Autodesk Inventor part; units mm, degrees
ref_plane "Work Plane1" through (0, 99.5, 0) normal (0, 1, 0) x (1, 0, 0)
ref_plane "Work Plane2" through (0, 0.5, 0) normal (0, -1, 0) x (1, 0, 0)
ref_plane "YZ Plane" through (0, 0, 0) normal (1, 0, 0) x (0, 1, 0)
sketch "Sketch1" plane through (0, 0, 0) normal (0, 1, 0) x (-1, 0, 0)
  circle A0 centre (0, 0) radius 1.4
  dimension "d0" = 2.8
extrude "Extrusion1" add sketch "Sketch1" along normal blind 100
ref_plane "Work Plane1" through (0, 99.5, 0) normal (0, 1, 0) x (1, 0, 0)
sketch "Sketch2" plane through (0, 99.5, 0) normal (0, 1, 0) x (1, 0, 0)
  line L0 (0, 0) -> (0, -1.5)
  line L1 (0, 0) -> (0, 1.5)
  dimension "d4" = 1.5
  dimension "d5" = 1.5
sketch "Sketch3" plane through (0, 0, 0) normal (1, 0, 0) x (0, 1, 0)
  line L0 (99.5, 0) -> (99.5, 1.5)
  line L1 (99.5, 0) -> (99.5, -1.5)
  line L2 (99.5, 1.5) -> (100.5, 1.5)
  line L3 (100.5, 1.5) -> (100.5, -1.5)
  line L4 (100.5, -1.5) -> (99.5, -1.5)
  line L5 (102, 1.659) -> (102, -3.2084)
  point P0 (0, 0)
  dimension "d6" = 1
  dimension "d7" = 2.5
revolve "Revolution1" add sketch "Sketch3" angle 360 about axis through (0, 102, 1.659) along (0, 0, -1)
ref_plane "Work Plane2" through (0, 0.5, 0) normal (0, -1, 0) x (1, 0, 0)
sketch "Sketch4" plane through (0, 0.5, 0) normal (0, -1, 0) x (1, 0, 0)
  line L0 (0, 0) -> (0, -2.1121)
  line L1 (3.5, -0.5) -> (3.5, 0.5)
  line L2 (3.5, 0.5) -> (0, 0.5)
  line L3 (3.5, -0.5) -> (0, -0.5)
  line L4 (-3.5, -0.5) -> (-3.5, 0.5)
  line L5 (-3.5, 0.5) -> (0, 0.5)
  line L6 (-3.5, -0.5) -> (0, -0.5)
  dimension "d12" = 3.5
  dimension "d13" = 1
extrude "Extrusion2" add sketch "Sketch4" along normal blind 9
sketch "Sketch5" plane through (3.5, 0.5, -0.5) normal (0, 0, -1) x (-1, 0, 0)
  line L0 (3.5, -0.5) -> (3.5, -9)
  line L1 (7, -9) -> (0, -9)
  line L2 (3.5, -9) -> (3.5, -5.5)
  line L3 (3.5, -9) -> (3.5, -9.0551)
  circle A0 centre (3.5, -5.5) radius 2
  dimension "d16" = 3.5
  dimension "d17" = 4
extrude "Extrusion3" add sketch "Sketch5" along normal blind 1.2
sketch "Sketch6" plane through (-3.5, 0.5, 0.5) normal (0, 0, 1) x (1, 0, 0)
  circle A0 centre (3.5, -5.5) radius 2
  point P0 (3.5, -0.5)
extrude "Extrusion4" add sketch "Sketch6" along normal blind 1.9
properties part number "101-05" material "Aluminum 6061"
CAD build for the part. Positions are in the model's coordinates, mm. A direction names the side the tool comes from. Round coordinates to 2 decimals unless told otherwise and drop trailing zeros. Loops run counter-clockwise (first coordinate to the right, second up) from the corner with the lowest first, then second, coordinate; pieces in that order, holes last. Notation, with made-up numbers: (-1, 53.5) - (18, 53.5) arc R28 ccw to (18, 87.5) - close; hole circle Ø8 at (54.5, 26). An arc over 180 degrees is marked (long way). Return JSON: item names as keys, results as strings. Group by question number.
Q1. Drill centre lines: line 1 along Y through (x, z) = (0, 0.9); line 2 along Y through (x, z) = (0, -0.15); line 3 along X through (y, z) = (102, -0.25). Where is each one in solid material? Low to high. Write a range as [from, to].
Q2. Flat gauge pins, fed straight in: pin 1 Ø2.5 at (x, y) = (-1, 101.5) entering from -Z; pin 2 Ø1.1 at (x, z) = (2.5, 0) entering from +Y; pin 3 Ø2 at (x, z) = (2, 1) entering from +Y. Where does each tip first touch, or does it go through?
Q3. Band-saw the part on A-A on x = 0. Give the cut face in (y, z), plus the area to 4 significant figures.
Q4. Band-saw the part on C-C on y = -5. Give the cut face in (x, z).
Q5. Tool access for faces 4 (the face through (1.4, 49.26, -0.06)), 5 (the face through (0, -7, 1)), 6 (the face through (-1, -3, -0.5)): list every direction of +Z, -Z, +X, -X, +Y, -Y with a clear straight run to the whole face (end or side of a thin tool).
Q6. Band-saw the part on B-B on y = 102. Give the cut face in (x, z), plus the area to 3 significant figures.
Q7. Two-plate mould, pull along X, no slides. Class faces 1 (the face through (-0.1, 104.5, 0)), 2 (the face through (2, 102, 1.5)), 3 (the face through (-1.265, 101.194, -0.021)): +X half, -X half, draft (parallel to the pull), parting line (faces both ways), or undercut.
Solutions:
{
 "1": {"line 1": "y = [-7, -3], [0, 100.5], [103.5, 104.5]", "line 2": "y = [-8.5, 100.5], [103.5, 104.5]", "line 3": "x = [-2.5, -1.5], [1.5, 2.5]"},
 "2": {"pin 1": "stops at z = -1.5", "pin 2": "stops at y = 103.56", "pin 3": "stops at y = 104.29"},
 "3": {"outline": "(-8.5, -0.5) - (-7, -0.5) - (-7, -1.7) - (-3, -1.7) - (-3, -0.5) - (0, -0.5) - (0, -1.4) - (99.5, -1.4) - (99.5, -1.5) - (100.5, -1.5) - (100.5, 1.5) - (99.5, 1.5) - (99.5, 1.4) - (0, 1.4) - (0, 0.5) - (-3, 0.5) - (-3, 2.4) - (-7, 2.4) - (-7, 0.5) - (-8.5, 0.5) - close; (103.5, -1.5) - (104.5, -1.5) - (104.5, 1.5) - (103.5, 1.5) - close", "area": "305.5 mm^2"},
 "4": {"outline": "(-3.5, -0.5) - (-2, -0.5) - (-2, -1.7) - (2, -1.7) - (2, -0.5) - (3.5, -0.5) - (3.5, 0.5) - (2, 0.5) - (2, 2.4) - (-2, 2.4) - (-2, 0.5) - (-3.5, 0.5) - close"},
 "5": {"face 4": "none", "face 5": "+Z", "face 6": "-Z"},
 "6": {"outline": "(-2.5, -1.5) - (-1.5, -1.5) - (-1.5, 1.5) - (-2.5, 1.5) - close; (1.5, -1.5) - (2.5, -1.5) - (2.5, 1.5) - (1.5, 1.5) - close", "area": "6.00 mm^2"},
 "7": {"face 1": "parting line", "face 2": "draft", "face 3": "undercut"}
}
